Geometry: final body of the model. Coordinates: model frame, mm. Face numbers are marked on the shaded views. A direction names the side the tool comes from. Round coordinates to 2 decimals unless told otherwise and drop trailing zeros. Order: outer loops, then holes, each group sorted by start corner. A loop starts at its lowest first (then second) coordinate and runs counter-clockwise, first axis right, second up. Notation, with made-up numbers: (67.25, 22) - (86.25, 22) arc R21 ccw to (86.25, 42) - close; hole circle Ø6 at (71, 0.5). An arc over 180 degrees is marked (long way). Put each result on its own line as item: value. Start each with the question number.
(1) Section B-B (z = -37.6). Output: boundary loops of the cut face in (x, y).
(2) Access query for the marked faces 4, 5 and 6. Directions: +Z, -Z, +X, -X, +Y, -Y. A direction counts if a zero-diameter tool reaches every point of the face in a straight line with its end or side. Return the directions, or none.
(3) Section C-C (z = 1.5). Output: boundary loops of the cut face in (x, y), and give its area (4 significant figures).
(4) Section D-D (y = 8). Count the separate pieces of the cut face and the enclosed holes in it, and give its area (3 significant figures).
(5) Section A-A (x = -28.05). Output: boundary loops of the cut face in (y, z), and give its area (3 significant figures).
(6) Pull-direction query (X, two-part tool) for the marked faces 1, 2 and 3; classes: released by +X, released by -X, zero draft, split by the parting line, or undercut.
(7) Material intervals for L1, parallel to X at y = -1.95, z = 37.6; L2, parallel to X at y = 4.5, z = 18; L3, parallel to Z at x = -14.5, y = 0.75, sorted ascending. Write a range as [from, to].
(8) Pin query (flat end, axial travel): P1, Ø8, axis at x = -4.5, y = 5.5, coming from the -Z side; P2, Ø3, axis at x = -23.5, y = 8.5, coming from the +Z side; P3, Ø8, axis at x = 25.5, z = 24.5, coming from the +Y side. Return the tip coordinate at first contact, or that it passes through.
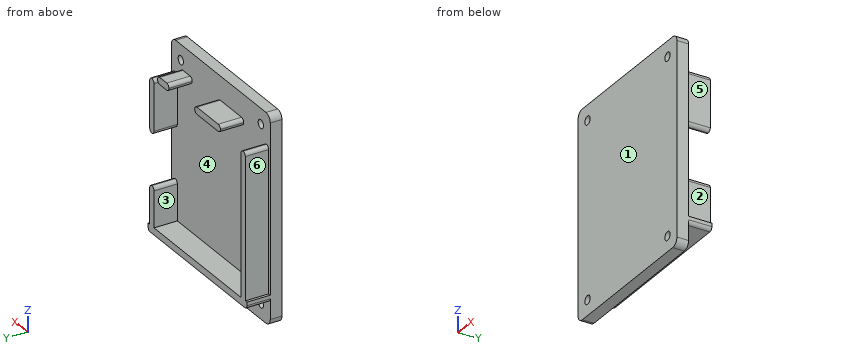
from build123d import *

# Parameters (mm, degrees)
SKETCH_1_W      = 69.3
SKETCH_1_H      = 88.4
SKETCH_1_R      = 1.85
EXTRUDE_1_DEPTH = 5
SKETCH_3_W      = 69.3
SKETCH_3_H      = 3
SKETCH_3_W_2    = 8
SKETCH_3_W_3    = 18
EXTRUDE_2_DEPTH = 10
SKETCH_4_W      = 3
SKETCH_4_H      = 62
SKETCH_4_H_2    = 17
SKETCH_4_H_3    = 23
EXTRUDE_3_DEPTH = 10
FILLET_1_R      = 3
FILLET_2_R      = 1.5
FILLET_3_R      = 1.5


with BuildPart() as part:
    # 草图1 → 凸台-拉伸1 (new body)
    with BuildSketch(Plane(origin=(0, 0, 0), x_dir=(1, 0, 0), z_dir=(0, 1, 0))):
        Rectangle(SKETCH_1_W, SKETCH_1_H)
        with Locations(Location((-28.05, 37.6, 0), (0, 0, 270))):
            Circle(SKETCH_1_R, mode=Mode.SUBTRACT)
        with Locations(Location((28.05, 37.6, 0), (0, 0, 90))):
            Circle(SKETCH_1_R, mode=Mode.SUBTRACT)
        with Locations(Location((28.05, -37.6, 0), (0, 0, 270))):
            Circle(SKETCH_1_R, mode=Mode.SUBTRACT)
        with Locations(Location((-28.05, -37.6, 0), (0, 0, 90))):
            Circle(SKETCH_1_R, mode=Mode.SUBTRACT)
    extrude(amount=-EXTRUDE_1_DEPTH)

    # 草图3 → 凸台-拉伸2 (add)
    with BuildSketch(Plane(origin=(0, 0, 0), x_dir=(1, 0, 0), z_dir=(0, 1, 0))):
        with Locations((0, 32.5)):
            Rectangle(SKETCH_3_W, SKETCH_3_H)
        with Locations((24.05, -32.5)):
            Rectangle(SKETCH_3_W_2, SKETCH_3_H)
        with Locations((-7.05, -32.5)):
            Rectangle(SKETCH_3_W_3, SKETCH_3_H)
    extrude(amount=EXTRUDE_2_DEPTH)

    # 草图4 → 凸台-拉伸3 (add)
    with BuildSketch(Plane(origin=(0, 0, 0), x_dir=(1, 0, 0), z_dir=(0, 1, 0))):
        with Locations((-32, 0)):
            Rectangle(SKETCH_4_W, SKETCH_4_H)
        with Locations((32, 22.5)):
            Rectangle(SKETCH_4_W, SKETCH_4_H_2)
        with Locations((32, -19.5)):
            Rectangle(SKETCH_4_W, SKETCH_4_H_3)
    extrude(amount=EXTRUDE_3_DEPTH)

    # 圆角1
    fillet_1_edges = [part.edges().sort_by_distance(p)[0] for p in [
        (34.65, -2.5, 44.2),
        (-34.65, -2.5, 44.2),
        (-34.65, -2.5, -44.2),
        (34.65, -2.5, -44.2),
    ]]
    fillet(fillet_1_edges, radius=FILLET_1_R)

    # 圆角2
    fillet_2_edges = [part.edges().sort_by_distance(p)[0] for p in [
        (20.05, 5, 34),
        (20.05, 5, 31),
        (28.05, 5, 31),
        (28.05, 5, 34),
        (-16.05, 5, 34),
        (-16.05, 5, 31),
        (1.95, 5, 34),
        (1.95, 5, 31),
    ]]
    fillet(fillet_2_edges, radius=FILLET_2_R - 0.0001)  # a hair under: the kernel refuses the full size

    # 圆角3
    fillet_3_edges = [part.edges().sort_by_distance(p)[0] for p in [
        (34.65, 5, -34),
        (-34.65, 5, -34),
        (-30.5, 5, 31),
        (-33.5, 5, 31),
        (33.5, 5, 31),
        (30.5, 5, 31),
        (33.5, 5, 8),
        (30.5, 5, 8),
        (33.5, 5, -14),
        (30.5, 5, -14),
    ]]
    fillet(fillet_3_edges, radius=FILLET_3_R - 0.0001)  # a hair under: the kernel refuses the full size


solid = part.part
Checks:
1. outline: (-34.65, -5) - (-29.9, -5) - (-29.9, 0) - (-34.65, 0) - close; (-26.2, -5) - (26.2, -5) - (26.2, 0) - (-26.2, 0) - close; (29.9, -5) - (34.65, -5) - (34.65, 0) - (29.9, 0) - close
2. face 4: +Y
2. face 5: +Z, +X, +Y
2. face 6: +Z, -X, +Y
3. outline: (-34.65, -5) - (34.65, -5) - (34.65, 0) - (-30.5, 0) - (-30.5, 10) - (-33.5, 10) - (-33.5, 0) - (-34.65, 0) - close
3. area: 376.5 mm²
4. separate pieces: 4
4. enclosed holes: 0
4. area: 583 mm²
5. outline: (-5, -44.2) - (0, -44.2) - (0, -39.45) - (-5, -39.45) - close; (-5, -35.75) - (0, -35.75) - (0, -34) - (10, -34) - (10, -31) - (0, -31) - (0, 35.75) - (-5, 35.75) - close; (-5, 39.45) - (0, 39.45) - (0, 44.2) - (-5, 44.2) - close
5. area: 435 mm²
6. face 1: zero draft
6. face 2: released by +X
6. face 3: undercut
7. L1: x = [-34.65, -29.9], [-26.2, 26.2], [29.9, 34.65]
7. L2: x = [-33.5, -30.5], [30.5, 33.5]
7. L3: z = [-34, -31], [31, 34]
8. P1: stops at z = -34
8. P2: stops at z = -31
8. P3: stops at y = 0
